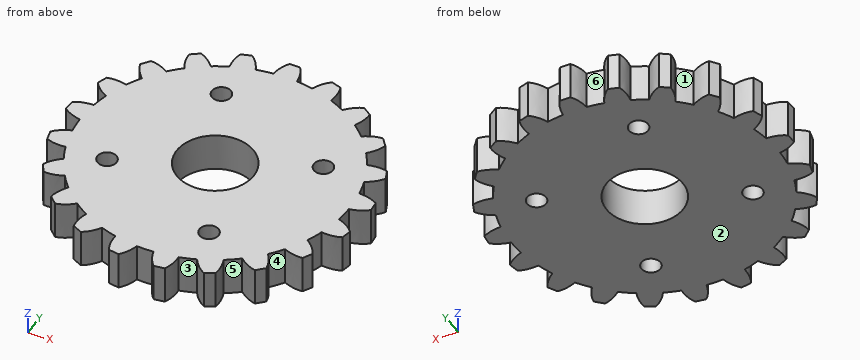
```python
from build123d import *

# Parameters (mm, degrees)
SKIZZE1_R                       = 10.5
AUFSATZ_LINEAR_AUSTRAGEN1_DEPTH = 3
AUFSATZ_LINEAR_AUSTRAGEN2_DEPTH = 3
KREISMUSTER1_COUNT              = 21
SKIZZE3_R                       = 0.75
SCHNITT_LINEAR_AUSTRAGEN1_DEPTH = 6.1
SKIZZE4_R                       = 3
SCHNITT_LINEAR_AUSTRAGEN2_DEPTH = 6.1


with BuildPart() as part:
    # Skizze1 → Aufsatz-Linear austragen1 (new body)
    with BuildSketch(Plane.XY):
        Circle(SKIZZE1_R)
    extrude(amount=AUFSATZ_LINEAR_AUSTRAGEN1_DEPTH)

    # Skizze2 → Aufsatz-Linear austragen2 (add)
    with BuildSketch(Plane.XY.offset(3)):
        with BuildLine():
            Line((0.920961993, 10.459532925), (-0.920961993, 10.459532925))
            add(Edge.make_bspline(
                [(-0.407740146, 11.911843377), (-0.824906562, 11.350994541), (-0.920961993, 10.459532925)],
                knots=[0, 0, 0, 1, 1, 1], degree=2))
            Line((-0.407740146, 11.911843377), (0.407740146, 11.911843377))
            add(Edge.make_bspline(
                [(0.407740146, 11.911843377), (0.824906562, 11.350994541), (0.920961993, 10.459532925)],
                knots=[0, 0, 0, 1, 1, 1], degree=2))
        make_face()
    aufsatz_linear_austragen2 = extrude(amount=-AUFSATZ_LINEAR_AUSTRAGEN2_DEPTH)

    # Kreismuster1: Aufsatz-Linear austragen2 ×21 about axis
    kreismuster1_axis = Axis((0, 0, 3), (0, 0, 1))
    for i in range(1, KREISMUSTER1_COUNT):
        add(aufsatz_linear_austragen2.rotate(kreismuster1_axis, i * 360 / KREISMUSTER1_COUNT))

    # Skizze3 → Schnitt-Linear austragen1 (cut)
    with BuildSketch(Plane.XY.offset(3)):
        with Locations((-3.085747028, 6.835800266)):
            Circle(SKIZZE3_R)
        with Locations((6.835800266, 3.085747028)):
            Circle(SKIZZE3_R)
        with Locations((-6.835800266, -3.085747028)):
            Circle(SKIZZE3_R)
        with Locations((3.085747028, -6.835800266)):
            Circle(SKIZZE3_R)
    extrude(amount=-SCHNITT_LINEAR_AUSTRAGEN1_DEPTH, mode=Mode.SUBTRACT)

    # Skizze4 → Schnitt-Linear austragen2 (cut)
    with BuildSketch(Plane.XY.offset(3)):
        Circle(SKIZZE4_R)
    extrude(amount=-SCHNITT_LINEAR_AUSTRAGEN2_DEPTH, mode=Mode.SUBTRACT)


solid = part.part
```
For this review, take the finished solid that the model builds, in its own axes (mm). Face numbers are marked on the shaded views. A direction names the side the tool comes from. Coordinates: 2 decimals unless noted, no trailing zeros. Order: outer loops, then holes, each group sorted by start corner. A loop starts at its lowest first (then second) coordinate and runs counter-clockwise, first axis right, second up. Notation, with made-up numbers: (54, -3) - (73, -3) arc R15 cw to (73, 20) - close; hole circle Ø6 at (32.25, 52.25). An arc over 180 degrees is marked (long way). Answer as a JSON object with one key per item and string values. Group by question number.
1. The part is to be moulded in two halves that separate along Y. For the marked faces 3, 4, 5 and 6, say which applies: pulls with the +Y half, pulls with the -Y half, needs draft (parallel to the pull), parting line crosses it, or undercut.
2. We need section C-C on y = 5.5. State the section outline as (x, z) points.
3. Clearance check with flat-ended pins moving along their axes: P1, Ø1.2, axis at x = 6.84, y = 3.09, coming from the +Z side; P2, Ø1.5, axis at y = 2.5, z = 1, coming from the -X side. State where each tip first meets the part, or that it passes through.
4. We need section B-B on z = 1.8. Give the number of separate pieces and of enclosed holes in the cut face, then the cut area to 3 significant figures.
5. For the marked faces 1 and 2, list the 3-axis set-ups (+Z, -Z, +X, -X, +Y, -Y) from which the entire face can be reached by the end or side of a thin tool; tool diameter is ignored.
6. We need section A-A on x = 0. State the section outline as (y, z) points, then the cut area to 3 significant figures.
7. For probe 1 along Y at (x, z) = (0, 2.1); probe 2 along Y at (x, z) = (6.5, 0.7); probe 3 along X at (y, z) = (-0.75, 0.5), list the stretches that pass through material, from the lowest coordinate up.
Final values:
{
 "1": {"face 3": "pulls with the -Y half", "face 4": "undercut", "face 5": "undercut", "face 6": "pulls with the +Y half"},
 "2": {"outline": "(-8.94, 0) - (8.94, 0) - (8.94, 3) - (-8.94, 3) - close"},
 "3": {"P1": "through", "P2": "x = -10.54"},
 "4": {"separate pieces": "1", "enclosed holes": "5", "area": "355 mm²"},
 "5": {"face 1": "+Z, -Z", "face 2": "-Z, +X, -X, +Y, -Y"},
 "6": {"outline": "(-10.5, 0) - (-3, 0) - (-3, 3) - (-10.5, 3) - close; (3, 0) - (11.91, 0) - (11.91, 3) - (3, 3) - close", "area": "49.2 mm²"},
 "7": {"probe 1": "-10.5 to -3, 3 to 11.91", "probe 2": "-8.35 to 2.42, 3.76 to 9.99", "probe 3": "-10.47 to -2.9, 2.9 to 10.47"}
}
